The listing builds one solid part. Answer for the finished solid, in the listing's coordinates (mm). Face numbers are marked on the shaded views. A direction names the side the tool comes from. Give positions to 0.01 mm unless a question says otherwise; leave off trailing zeros. Order: outer loops, then holes, each group sorted by start corner. A loop starts at its lowest first (then second) coordinate and runs counter-clockwise, first axis right, second up. Notation, with made-up numbers: (-8, 87) - (50, 87) arc R7 cw to (50, 93) - close; hole circle Ø11 at (44.5, -20). An arc over 180 degrees is marked (long way). Answer as a JSON object with one key per item and string values. Group by question number.
Q1. Given pin 1 (2 mm diameter, centred on y = 1.5, z = 8.5, fed in from +X); pin 2 (8 mm diameter, centred on x = -18.3, z = -5, fed in from +Y); pin 3 (3 mm diameter, centred on y = -5.5, z = 10, fed in from +X); pin 4 (4 mm diameter, centred on x = -24, y = 1, fed in from -Z), each flat-ended and moving along its own axis, determine where each tip first touches the part or whether it passes through.
Q2. A cutting plane is placed at B-B, the plane y = -27. Give the vertices of the cut face in (x, z).
Q3. A cutting plane is placed at D-D, the plane y = -1. Give the vertices of the cut face in (x, z).
Q4. Consider line 1 (X direction, y = -7, z = 3); line 2 (X direction, y = -23, z = 11.5); line 3 (X direction, y = 11.25, z = -5). Determine where each line is inside the solid, lowest interval first.
Q5. A cutting plane is placed at A-A, the plane x = 0. Give the vertices of the cut face in (y, z).
Q6. A cutting plane is placed at C-C, the plane z = -5. Give the vertices of the cut face in (x, y).
Q7. For the marked faces 1, 2, 3, 4 and 5, determine the directions among +Z, -Z, +X, -X, +Y, -Y from which every point of the face is accessible in a straight line to the end or side of a thin tool.
Q8. The mould has two halves that part along X. Classify the marked faces 6, 7 and 8: released by +X, released by -X, zero draft, split by the parting line, or undercut.
from build123d import *

# Parameters (mm, degrees)
BOSS_EXTRUDE1_DEPTH = 17
BOSS_EXTRUDE2_START = -17
BOSS_EXTRUDE2_DEPTH = 2
SKETCH3_R           = 2
CUT_EXTRUDE2_DEPTH  = 53.410576235
SKETCH4_R           = 5.334569818
CUT_EXTRUDE3_DEPTH  = 14
SKETCH5_R           = 2
BOSS_EXTRUDE3_DEPTH = 3
CUT_EXTRUDE4_DEPTH  = 57.452356029
CHAMFER2_SIZE       = 10
FILLET1_R           = 15
FILLET2_R           = 15
SKETCH7_R           = 5
CUT_EXTRUDE6_DEPTH  = 62.913395196


with BuildPart() as part:
    # Sketch1 → Boss-Extrude1 (new body)
    with BuildSketch(Plane.XY):
        with BuildLine():
            Line((38.034569818, 17.9), (3.805259518, 17.9))
            ThreePointArc((3.805259518, 17.9), (14.221924082, 11.51637423), (18.3, 0))
            Line((18.3, 0), (18.3, -10))
            ThreePointArc((18.3, -10), (0, -28.3), (-18.3, -10))
            Line((-18.3, -10), (-18.3, 0))
            ThreePointArc((-18.3, 0), (-14.221924082, 11.51637423), (-3.805259518, 17.9))
            Line((-3.805259518, 17.9), (-38.034569818, 17.9))
            Line((-38.034569818, 17.9), (-27.7, 0))
            Line((-27.7, 0), (-27.7, -12.5))
            Line((-27.7, -12.5), (-15.801197979, -25.018726392))
            ThreePointArc((-15.801197979, -25.018726392), (0, -31.8), (15.801197979, -25.018726392))
            Line((15.801197979, -25.018726392), (27.7, -12.5))
            Line((27.7, -12.5), (27.7, 0))
            Line((27.7, 0), (38.034569818, 17.9))
        make_face()
        with BuildLine():
            Line((23.7, 0), (23.7, -10))
            ThreePointArc((23.7, -10), (22, -11.7), (20.3, -10))
            Line((20.3, -10), (20.3, 0))
            ThreePointArc((20.3, 0), (22, 1.7), (23.7, 0))
        make_face(mode=Mode.SUBTRACT)
        with BuildLine():
            Line((-23.7, 0), (-23.7, -10))
            ThreePointArc((-23.7, -10), (-22, -11.7), (-20.3, -10))
            Line((-20.3, -10), (-20.3, 0))
            ThreePointArc((-20.3, 0), (-22, 1.7), (-23.7, 0))
        make_face(mode=Mode.SUBTRACT)
    extrude(amount=BOSS_EXTRUDE1_DEPTH)

    # Sketch2 → Boss-Extrude2 (add)
    with BuildSketch(Plane.XY.offset(17).offset(BOSS_EXTRUDE2_START)):
        Polygon((38.034569818, 17.9), (-38.034569818, 17.9), (-30.586751346, 5), (30.586751346, 5), align=None)
    extrude(amount=BOSS_EXTRUDE2_DEPTH)

    # Sketch3 → Cut-Extrude2 (cut, through all)
    with BuildSketch(Plane(origin=(0, 0, 0), x_dir=(1, 0, 0), z_dir=(0, 1, 0))):
        with Locations(Location((32.7, -8.5, 0), (0, 0, 180))):
            Circle(SKETCH3_R)
    cut_extrude2 = extrude(amount=CUT_EXTRUDE2_DEPTH, mode=Mode.SUBTRACT)

    # Sketch4 → Cut-Extrude3 (cut)
    with BuildSketch(Plane(origin=(0, 0, 0), x_dir=(1, 0, 0), z_dir=(0, 1, 0))):
        with Locations((32.7, -8.5)):
            Circle(SKETCH4_R)
    cut_extrude3 = extrude(amount=CUT_EXTRUDE3_DEPTH, mode=Mode.SUBTRACT)

    # Sketch5 → Boss-Extrude3 (add)
    with BuildSketch(Plane(origin=(0, 17.9, 0), x_dir=(1, 0, 0), z_dir=(0, 1, 0))):
        Polygon((-38.034569818, 0), (-23.753089751, 10), (0, 10), (0, 0), align=None)
        with Locations(Location((-18.3, 5, 0), (0, 0, 180))):
            Circle(SKETCH5_R, mode=Mode.SUBTRACT)
    boss_extrude3 = extrude(amount=-BOSS_EXTRUDE3_DEPTH)

    # Sketch6 → Cut-Extrude4 (cut, through all)
    with BuildSketch(Plane(origin=(0, 0, -10), x_dir=(-1, 0, 0), z_dir=(0, 0, -1))):
        Polygon((36.302519011, 14.9), (38.034569818, 17.9), (38.034569818, 14.9), align=None)
    cut_extrude4 = extrude(amount=-CUT_EXTRUDE4_DEPTH, mode=Mode.SUBTRACT)

    # Mirror2: Cut-Extrude2, Cut-Extrude3, Boss-Extrude3 across plane
    add(cut_extrude2.mirror(Plane(origin=(0, 14.9, -10), x_dir=(0, 0, 1), z_dir=(1, 0, 0))), mode=Mode.SUBTRACT)
    add(cut_extrude3.mirror(Plane(origin=(0, 14.9, -10), x_dir=(0, 0, 1), z_dir=(1, 0, 0))), mode=Mode.SUBTRACT)
    add(boss_extrude3.mirror(Plane(origin=(0, 14.9, -10), x_dir=(0, 0, 1), z_dir=(1, 0, 0))))

    # Mirror3: Cut-Extrude2, Cut-Extrude3, Cut-Extrude4 across plane
    add(cut_extrude2.mirror(Plane(origin=(0, 0, 0), x_dir=(0, 0, 1), z_dir=(1, 0, 0))), mode=Mode.SUBTRACT)
    add(cut_extrude3.mirror(Plane(origin=(0, 0, 0), x_dir=(0, 0, 1), z_dir=(1, 0, 0))), mode=Mode.SUBTRACT)
    add(cut_extrude4.mirror(Plane(origin=(0, 0, 0), x_dir=(0, 0, 1), z_dir=(1, 0, 0))), mode=Mode.SUBTRACT)

    # Chamfer2
    # the kernel refuses this chamfer: 10 mm, written as the material it adds along each edge
    with BuildSketch(Plane(origin=(-62.019348891, 14.9, 0), x_dir=(0, 0.027495876610586317, -0.9996219169112968), z_dir=(1, 0, 0))) as chamfer2_piece_1_section:
        Polygon((CHAMFER2_SIZE * 0.999621916911, -CHAMFER2_SIZE * 0.0274958766106), (-CHAMFER2_SIZE * 0.0274958766106, -CHAMFER2_SIZE * 0.999621916911), (0, 0), align=None)
    chamfer2_piece_1 = extrude(amount=124.038697781, mode=Mode.PRIVATE)
    chamfer2_piece_1 = chamfer2_piece_1 - Plane(origin=(18.3, 11.716008288, -5), x_dir=(1, 0, 0), z_dir=(0, 1, 0)) * Cylinder(2, 289, mode=Mode.PRIVATE)
    chamfer2_piece_1 = chamfer2_piece_1 - Plane(origin=(-18.3, 11.716008288, -5), x_dir=(-1, 0, 0), z_dir=(0, 1, 0)) * Cylinder(2, 289, mode=Mode.PRIVATE)
    chamfer2_piece_1 = split(chamfer2_piece_1, bisect_by=Plane(origin=(-4.622195202, 11.716008288, -29.868588423), z_dir=(-0.5735764363510418, 0, 0.819152044288995)), keep=Keep.TOP, mode=Mode.PRIVATE)
    chamfer2_piece_1 = split(chamfer2_piece_1, bisect_by=Plane(origin=(-26.779856727, 11.716008288, -7.880634947), z_dir=(0.5735764363510418, 0, 0.819152044288995)), keep=Keep.TOP, mode=Mode.PRIVATE)
    chamfer2_piece_1 = split(chamfer2_piece_1, bisect_by=Plane(origin=(-31.697953242, 6.924658142, -3.052401614), z_dir=(0.8660254037844364, 0.500000000000004, 0)), keep=Keep.TOP, mode=Mode.PRIVATE)
    chamfer2_piece_1 = chamfer2_piece_1 - Plane(origin=(0, 0, -3.052401614), x_dir=(-1, 0, 0), z_dir=(0, 0, -1)) * Cylinder(18.3, 289, mode=Mode.PRIVATE)
    chamfer2_piece_1 = split(chamfer2_piece_1, bisect_by=Plane(origin=(19.998407566, -13.339549394, -3.052401614), z_dir=(-0.8660254037844365, 0.5000000000000038, 0)), keep=Keep.TOP, mode=Mode.PRIVATE)
    add(chamfer2_piece_1)
    with BuildSketch(Plane(origin=(-62.019348891, 14.9, 0), x_dir=(0, 0.027495876610586317, -0.9996219169112968), z_dir=(1, 0, 0))) as chamfer2_piece_2_section:
        Polygon((CHAMFER2_SIZE * 0.999621916911, -CHAMFER2_SIZE * 0.0274958766106), (-CHAMFER2_SIZE * 0.0274958766106, -CHAMFER2_SIZE * 0.999621916911), (0, 0), align=None)
    chamfer2_piece_2 = extrude(amount=124.038697781, mode=Mode.PRIVATE)
    chamfer2_piece_2 = split(chamfer2_piece_2, bisect_by=Plane(origin=(0, 5, -3.178355845), z_dir=(0, 1, 0)), keep=Keep.TOP, mode=Mode.PRIVATE)
    chamfer2_piece_2 = chamfer2_piece_2 & Plane(origin=(0, 0, -3.178355845), x_dir=(-1, 0, 0), z_dir=(0, 0, -1)) * Cylinder(18.3, 289, mode=Mode.PRIVATE)
    add(chamfer2_piece_2)

    # Fillet1
    fillet1_edges = [part.edges().sort_by_distance(p)[0] for p in [
        (27.7, -12.5, 8.5),
        (-27.7, -12.5, 8.5),
    ]]
    fillet(fillet1_edges, radius=FILLET1_R)

    # Fillet2
    fillet2_edges = [part.edges().sort_by_distance(p)[0] for p in [
        (27.7, 0, 13.67973587),
        (27.7, 0, 3.32026413),
        (-27.7, 0, 13.67973587),
        (-27.7, 0, 3.32026413),
    ]]
    fillet(fillet2_edges, radius=FILLET2_R)

    # Sketch7 → Cut-Extrude6 (cut, through all)
    with BuildSketch(Plane.XZ.offset(-14)):
        with Locations((-18.3, -5)):
            Circle(SKETCH7_R)
    cut_extrude6 = extrude(amount=CUT_EXTRUDE6_DEPTH, mode=Mode.SUBTRACT)

    # Mirror4: Cut-Extrude6 across plane
    add(cut_extrude6.mirror(Plane(origin=(0, 0, 0), x_dir=(0, 0, 1), z_dir=(1, 0, 0))), mode=Mode.SUBTRACT)


solid = part.part
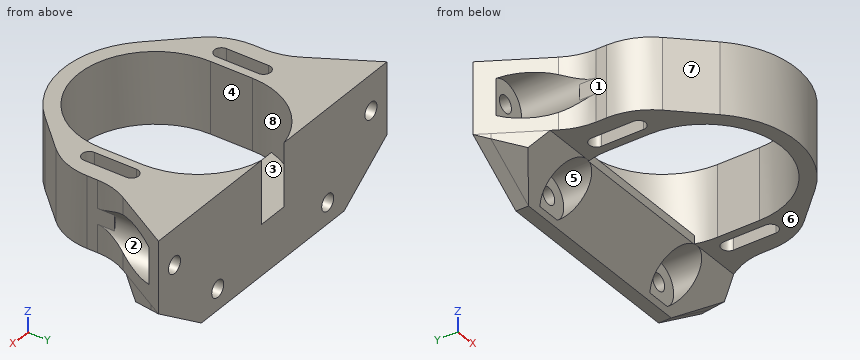
Reply:
{
 "1": {"pin 1": "stops at x = 27.46", "pin 2": "stops at y = 17.9", "pin 3": "stops at x = 27.7", "pin 4": "stops at z = 0"},
 "2": {"outline": "(-13.65, 0) - (-6.77, 0) - (-6.77, 17) - (-13.65, 17) - close; (6.77, 0) - (13.65, 0) - (13.65, 17) - (6.77, 17) - close"},
 "3": {"outline": "(-28.01, 0) - (-23.7, 0) - (-23.7, 17) - (-28.01, 17) - (-28.01, 11.04) arc R5.33 cw to (-27.7, 10.36) - (-27.7, 6.64) arc R5.33 cw to (-28.01, 5.96) - close; (-20.3, 0) - (-18.3, 0) - (-18.3, 17) - (-20.3, 17) - close; (18.3, 0) - (20.3, 0) - (20.3, 17) - (18.3, 17) - close; (23.7, 0) - (28.01, 0) - (28.01, 5.96) arc R5.33 cw to (27.7, 6.64) - (27.7, 10.36) arc R5.33 cw to (28.01, 11.04) - (28.01, 17) - (23.7, 17) - close"},
 "4": {"line 1": "x = -27.69 to -23.7, -20.3 to -18.3, 18.3 to 20.3, 23.7 to 27.69", "line 2": "x = -17.72 to -12.88, 12.88 to 17.72", "line 3": "x = -30.89 to -23.3, -13.3 to 13.3, 23.3 to 30.89"},
 "5": {"outline": "(-31.8, 0) - (-28.3, 0) - (-28.3, 17) - (-31.8, 17) - close; (5, -0.1) - (14.9, -10) - (17.9, -10) - (17.9, 2) - (5, 2) - close"},
 "6": {"outline": "(-30.89, 9.9) - (-23.3, 9.9) - (-23.3, 14) - (-20.3, 14) - (-20.3, 17.9) - (-30.89, 17.9) - close; (-16.3, 14) - (-13.3, 14) - (-13.3, 9.9) - (13.3, 9.9) - (13.3, 14) - (16.3, 14) - (16.3, 17.9) - (-16.3, 17.9) - close; (20.3, 14) - (23.3, 14) - (23.3, 9.9) - (30.89, 9.9) - (30.89, 17.9) - (20.3, 17.9) - close"},
 "7": {"face 1": "-X, -Y", "face 2": "none", "face 3": "+Z", "face 4": "+Z, -Z", "face 5": "-Y"},
 "8": {"face 6": "zero draft", "face 7": "released by -X", "face 8": "undercut"}
}
